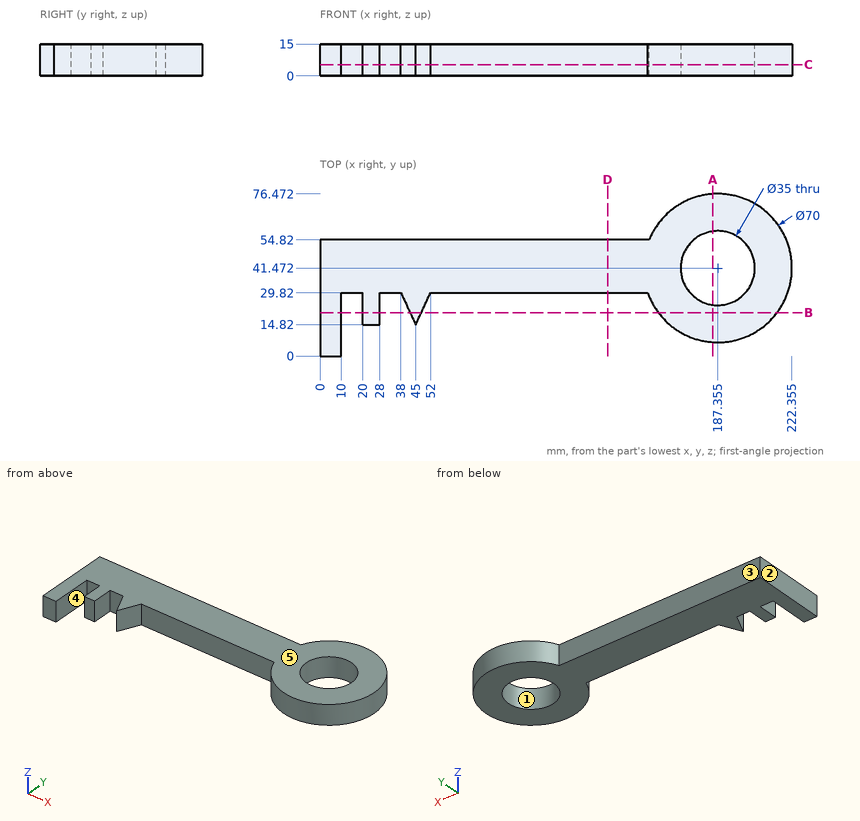
The drawing under review shows one solid part. Ordinate dimensions are in mm from its lowest x, y, z. A direction names the side the tool comes from. Coordinates: 2 decimals unless noted, no trailing zeros. Write each loop counter-clockwise with the first axis right and the second up, starting at its lowest first coordinate (ties: lowest second). Pieces come first, ordered by that corner, then holes. Notation, with made-up numbers: M 17.5,22.5 L 29.5,22.5 A21 ccw 29.5,35.5 Z; hole C -18.75,62 d11. An arc over 180 degrees is marked long. Answer as a JSON object with one key per item and string values.
Item 1: Insertion check: pin 1 Ø1 at (x, z) = (133, 4) entering from +Y; pin 2 Ø1.5 at (y, z) = (20.5, 10) entering from +X; pin 3 Ø9 at (x, z) = (22.5, 4) entering from -Y. Each pin has a flat end and moves straight along its axis. Give the tip position at first contact, or say it passes through.
Outcome:
{"pin 1": "y = 54.82", "pin 2": "x = 215.92", "pin 3": "y = 14.82"}
Item 2: Add section B-B, the plane y = 20.5. Give the boundary of the cut face in (x, z), and give its area (3 significant figures).
Outcome:
{"outline": "M 0,0 L 10,0 L 10,15 L 0,15 Z; M 20,0 L 28,0 L 28,15 L 20,15 Z; M 42.35,0 L 47.65,0 L 47.65,15 L 42.35,15 Z; M 159.33,0 L 215.38,0 L 215.38,15 L 159.33,15 Z", "area": "1,190 mm²"}
Item 3: Add section C-C, the plane z = 5.25. Give the boundary of the cut face in (x, y) (1 decimal).
Outcome:
{"outline": "M 0,0 L 10,0 L 10,29.8 L 20,29.8 L 20,14.8 L 28,14.8 L 28,29.8 L 38,29.8 L 45,14.8 L 52,29.8 L 154.4,29.8 A35 ccw long 155,54.8 L 0,54.8 Z; hole C 187.4,41.5 d35"}
Item 4: Draft analysis for pull direction X (two halves, no side actions). For the marked faces 1, 2 and 3, state which applies: pulls with the +X half, pulls with the -X half, needs draft (parallel to the pull), parting line crosses it, or undercut.
Outcome:
{"face 1": "undercut", "face 2": "pulls with the -X half", "face 3": "needs draft"}
Item 5: Machinability: for the marked faces 4 and 5, which of the approach directions +Z, -Z, +X, -X, +Y, -Y give a long, thin tool a straight path to every point of the face, cutting with its end or side? Answer none if there is none.
Outcome:
{"face 4": "+Z, -Z, -Y", "face 5": "+Z, +X, -X, +Y, -Y"}
Item 6: Add section D-D, the plane x = 135.5. Give the boundary of the cut face in (y, z).
Outcome:
{"outline": "M 29.82,0 L 54.82,0 L 54.82,15 L 29.82,15 Z"}
Item 7: Add section A-A, the plane x = 185. Give the boundary of the cut face in (y, z), and give its area (3 significant figures).
Outcome:
{"outline": "M 6.55,0 L 24.13,0 L 24.13,15 L 6.55,15 Z; M 58.81,0 L 76.39,0 L 76.39,15 L 58.81,15 Z", "area": "527 mm²"}
Item 8: Wall thickness on probe 1 along X at (y, z) = (28.5, 10.25) (1 decimal); probe 2 along X at (y, z) = (27.5, 11) (1 decimal); probe 3 along Y at (x, z) = (35, 8.75): over which ranges is each line inside the solid? List them lowest first.
Outcome:
{"probe 1": "0 to 10, 20 to 28, 38.6 to 51.4, 154.8 to 175.6, 199.1 to 219.9", "probe 2": "0 to 10, 20 to 28, 39.1 to 50.9, 155.3 to 176.8, 197.9 to 219.4", "probe 3": "29.82 to 54.82"}
